Build history of the part. All positions in model axes, mm. A direction names the side the tool comes from. Give positions to 0.01 mm unless a question says otherwise; leave off trailing zeros. Write each loop counter-clockwise with the first axis right and the second up, starting at its lowest first coordinate (ties: lowest second). Pieces come first, ordered by that corner, then holes. Notation, with made-up numbers: M 30.5,-21 L 48.5,-21 A18 cw 48.5,11 Z; hole C 67.25,40 d11. An arc over 180 degrees is marked long. Return JSON: item names as keys, results as strings. Group by question number.
Q1. Wall check: probe 1 along Y at (x, z) = (-5, 4.5); probe 2 along Z at (x, y) = (-42.5, 1.75). Give the ranges that are in metal, low to high.
Q2. Tool access for faces 5 (the flat face through (-34, 0, 34)), 6 (the flat face through (-34, 15, 1.588)): list every direction of +Z, -Z, +X, -X, +Y, -Y with a clear straight run to the whole face (end or side of a thin tool).
Q3. Band-saw the part on C-C, the plane x = -64. Give the cut face in (y, z), then the cut area to 3 significant figures.
Q4. Flat gauge pins, fed straight in: pin 1 Ø12 at (x, z) = (-16.5, 67) entering from +Y; pin 2 Ø5.5 at (x, y) = (-38.1, 12.7) entering from +Z; pin 3 Ø10 at (x, y) = (-63.5, 12.7) entering from +Z. Where does each tip first touch, or does it go through?
Q5. Band-saw the part on D-D, the plane x = -38.1. Give the cut face in (y, z) (1 decimal), then the cut area to 3 significant figures.
Q6. Band-saw the part on B-B, the plane y = 12.7. Count the separate pieces of the cut face and the enclosed holes in it, then the cut area to 3 significant figures.
Q7. Pull direction Y, two halves, no side cores. Call faces 1 (the flat face through (-34, 1.588, 37)), 2 (the cylindrical face through (-66.53, 13.65, 0.78)), 3 (the flat face through (-34, 14, 0)), 4 (the cylindrical face through (-34.93, 12.84, 0.78)): +Y half, -Y half, draft (parallel to the pull), parting line (faces both ways), or undercut.
Autodesk Inventor part; units mm, degrees
ref_plane "YZ Plane" through (0, 0, 0) normal (1, 0, 0) x (0, 1, 0)
ref_plane "XZ Plane" through (0, 0, 0) normal (0, 1, 0) x (-1, 0, 0)
ref_plane "XY Plane" through (0, 0, 0) normal (0, 0, 1) x (1, 0, 0)
sketch "Sketch1" plane through (0, 0, 0) normal (0, 1, 0) x (-1, 0, 0)
  line L0 (69.85, 88.9) -> (0, 88.9)
  line L1 (0, 88.9) -> (0, 0)
  line L2 (0, 0) -> (69.85, 0)
  line L3 (69.85, 0) -> (69.85, 88.9)
extrude "Extrusion1" add sketch "Sketch1" along normal blind 1.5875
chamfer "Chamfer1" distance 14.2875 angle 45 1 edges at (-69.85, 0.7937, 88.9)
chamfer "Chamfer2" distance 14.2875 angle 45 1 edges at (0, 0.7937, 88.9)
sketch "Sketch2" plane through (0, 0, 0) normal (0, 0, -1) x (-1, 0, 0)
  line L0 (69.85, 26.9875) -> (0, 26.9875)
  line L1 (0, 26.9875) -> (0, 0)
  line L2 (0, 0) -> (69.85, 0)
  line L3 (69.85, 0) -> (69.85, 26.9875)
sketch "Sketch3" plane through (0, 0, 0) normal (1, 0, 0) x (0, 0, -1)
  line L0 (0, 0) -> (-1.5875, 0)
  line L1 (-1.5875, 0) -> (-1.5875, 1.5875)
  line L2 (-1.5875, 1.5875) -> (0, 1.5875)
  line L3 (0, 1.5875) -> (0, 0)
  dimension "d8" = 1.5875
  dimension "d9" = 1.5875
extrude "Extrusion2" cut sketch "Sketch3" against normal blind 69.85
extrude "Extrusion3" add sketch "Sketch2" against normal blind 1.5875
fillet "Fillet1" radius 0.7937 1 edges at (-34.925, 1.5875, 1.5875)
fillet "Fillet2" radius 0.7937 1 edges at (-34.925, 0, 0)
sketch "Sketch4" plane through (0, 0, 0) normal (0, 0, -1) x (-1, 0, 0)
  circle A0 centre (12.7, 12.7) radius 3.175
  point P0 (0, 0)
  dimension "d16" = 6.35
extrude "Extrusion4" cut sketch "Sketch4" against normal blind 1.5875
sketch "Sketch5" plane through (0, 0, 0) normal (0, 0, -1) x (-1, 0, 0)
  circle A0 centre (63.5, 12.7) radius 3.175
  point P0 (0, 0)
  dimension "d19" = 6.35
extrude "Extrusion5" cut sketch "Sketch5" against normal blind 1.5875
sketch "Sketch6" plane through (0, 0, 0) normal (0, 0, -1) x (-1, 0, 0)
  circle A0 centre (38.1, 12.7) radius 3.175
  point P0 (0, 0)
  dimension "d22" = 6.35
extrude "Extrusion6" cut sketch "Sketch6" against normal blind 1.5875
sketch "Sketch7" plane through (0, 0, 0) normal (0, -1, 0) x (1, 0, 0)
  circle A0 centre (-34.925, 50.8) radius 12.7
  point P0 (0, 0)
  dimension "d25" = 25.4
extrude "Extrusion7" cut sketch "Sketch7" against normal blind 1.5875
properties part number "alignmentWheelsBarP2"
From the geometry:
{
 "1": {"probe 1": "y = 0 to 1.59", "probe 2": "z = 0 to 1.9"},
 "2": {"face 5": "+Z, -Z, +X, -X, -Y", "face 6": "+Z, +X, -X, +Y"},
 "3": {"outline": "M 0,0.79 A0.79 ccw 0.79,0 L 9.56,0 L 9.56,1.59 L 2.38,1.59 A0.79 cw 1.59,2.38 L 1.59,80.46 L 0,80.46 Z; M 15.84,0 L 26.99,0 L 26.99,1.59 L 15.84,1.59 Z", "area": "158 mm^2"},
 "4": {"pin 1": "stops at y = 1.59", "pin 2": "passes through", "pin 3": "stops at z = 1.59"},
 "5": {"outline": "M 0,0.8 A0.8 ccw 0.8,0 L 9.5,0 L 9.5,1.6 L 2.4,1.6 A0.8 cw 1.6,2.4 L 1.6,38.5 L 0,38.5 Z; M 0,63.1 L 1.6,63.1 L 1.6,88.9 L 0,88.9 Z; M 15.9,0 L 27,0 L 27,1.6 L 15.9,1.6 Z", "area": "132 mm^2"},
 "6": {"separate pieces": "4", "enclosed holes": "0", "area": "80.6 mm^2"},
 "7": {"face 1": "+Y half", "face 2": "undercut", "face 3": "draft", "face 4": "undercut"}
}
